Source: CAD feature listing. Evaluate the final solid. Frame: model axes, mm. A direction names the side the tool comes from. Give positions to 0.01 mm unless a question says otherwise; leave off trailing zeros. Write each loop counter-clockwise with the first axis right and the second up, starting at its lowest first coordinate (ties: lowest second). Pieces come first, ordered by that corner, then holes. Notation, with made-up numbers: (25.25, -37.75) -> (42.25, -37.75) arc R22 cw to (42.25, -25.75) -> close; hole circle Ø7 at (-29, 19.5). An arc over 180 degrees is marked (long way). Answer as a JSON object with one key per item and string values. Group by question number.
Item 1: Access query for faces 1 (the face through (0, 1, 13.5)), 2 (the face through (12.5, 1, -3)), 3 (the face through (13, 9, 0)), 4 (the face through (11.93, 10.01, 11.9)). Directions: +Z, -Z, +X, -X, +Y, -Y. A direction counts if a zero-diameter tool reaches every point of the face in a straight line with its end or side. Return the directions, or none.
Item 2: Section query C-C on x = -3.75. Return the cut outline in (y, z), plus the area to 3 significant figures.
Item 3: Section query D-D on z = -4.5. Return the cut outline in (x, y).
Item 4: First-contact query: pin 1 Ø0.6 at (y, z) = (1.5, -6.5) entering from -X; pin 2 Ø0.6 at (x, y) = (-1.5, 0.5) entering from -Z; pin 3 Ø2 at (y, z) = (0.5, -1.5) entering from +X; pin 4 Ø1.6 at (y, z) = (1.5, 10.5) entering from -X. Flat tips, straight axial feed; report the tip coordinate or a pass-through.
Item 5: Section query B-B on x = 7. Return the cut outline in (y, z).
Item 6: Section query A-A on z = 7.25. Return the cut outline in (x, y), plus the area to 3 significant figures.
Item 7: Ray query, probe 1 along X at (y, z) = (10, -5); probe 2 along Z at (x, y) = (4, 0.75); probe 3 along Z at (x, y) = (8.75, 1.5). Return the intervals inside material, ascending. Write a range as from..to.
from build123d import *

# Parameters (mm, degrees)
SKETCH1_W           = 29
SKETCH1_H           = 29
BOSS_EXTRUDE1_DEPTH = 11
CUT_EXTRUDE1_DEPTH  = 2
SKETCH3_W           = 29
SKETCH3_H           = 29
SKETCH3_W_2         = 25
SKETCH3_H_2         = 18
CUT_EXTRUDE2_DEPTH  = 2
SKETCH4_W           = 9.666666666
SKETCH4_H           = 4
BOSS_EXTRUDE2_DEPTH = 2


with BuildPart() as part:
    # Sketch1 → Boss-Extrude1 (new body)
    with BuildSketch(Plane(origin=(0, 0, 0), x_dir=(1, 0, 0), z_dir=(0, 1, 0))):
        Rectangle(SKETCH1_W, SKETCH1_H)
    extrude(amount=BOSS_EXTRUDE1_DEPTH)

    # Sketch2 → Cut-Extrude1 (cut)
    with BuildSketch(Plane(origin=(0, 11, 0), x_dir=(1, 0, 0), z_dir=(0, 1, 0))):
        with BuildLine():
            Line((-10.5, 17.5), (10.5, 17.5))
            ThreePointArc((10.5, 17.5), (15.449747468, 15.449747468), (17.5, 10.5))
            Line((17.5, 10.5), (17.5, -10.5))
            ThreePointArc((17.5, -10.5), (15.449747468, -15.449747468), (10.5, -17.5))
            Line((10.5, -17.5), (-10.5, -17.5))
            ThreePointArc((-10.5, -17.5), (-15.449747468, -15.449747468), (-17.5, -10.5))
            Line((-17.5, -10.5), (-17.5, 10.5))
            ThreePointArc((-17.5, 10.5), (-15.449747468, 15.449747468), (-10.5, 17.5))
        make_face()
        with BuildLine():
            Line((-10.5, 12.5), (10.5, 12.5))
            ThreePointArc((10.5, 12.5), (11.914213562, 11.914213562), (12.5, 10.5))
            Line((12.5, 10.5), (12.5, -10.5))
            ThreePointArc((12.5, -10.5), (11.914213562, -11.914213562), (10.5, -12.5))
            Line((10.5, -12.5), (-10.5, -12.5))
            ThreePointArc((-10.5, -12.5), (-11.914213562, -11.914213562), (-12.5, -10.5))
            Line((-12.5, -10.5), (-12.5, 10.5))
            ThreePointArc((-12.5, 10.5), (-11.914213562, 11.914213562), (-10.5, 12.5))
        make_face(mode=Mode.SUBTRACT)
    extrude(amount=-CUT_EXTRUDE1_DEPTH, mode=Mode.SUBTRACT)

    # Sketch3 → Cut-Extrude2 (cut)
    with BuildSketch(Plane(origin=(0, 0, 0), x_dir=(-1, 0, 0), z_dir=(0, -1, 0))):
        Rectangle(SKETCH3_W, SKETCH3_H)
        with Locations((0, 3.5)):
            Rectangle(SKETCH3_W_2, SKETCH3_H_2, mode=Mode.SUBTRACT)
    extrude(amount=-CUT_EXTRUDE2_DEPTH, mode=Mode.SUBTRACT)

    # Sketch4 → Boss-Extrude2 (add)
    with BuildSketch(Plane.XZ.offset(-2)):
        with Locations((0, 11.5)):
            Rectangle(SKETCH4_W, SKETCH4_H)
    extrude(amount=BOSS_EXTRUDE2_DEPTH)


solid = part.part
Worked answers:
{
 "1": {"face 1": "+Z, +X, -X, -Y", "face 2": "+Z, -Z, +X, -Y", "face 3": "+Y", "face 4": "+Z, +X, +Y"},
 "2": {"outline": "(0, -12.5) -> (2, -12.5) -> (2, -14.5) -> (9, -14.5) -> (9, -12.5) -> (11, -12.5) -> (11, 12.5) -> (9, 12.5) -> (9, 14.5) -> (2, 14.5) -> (2, 13.5) -> (0, 13.5) -> (0, 9.5) -> (2, 9.5) -> (2, 5.5) -> (0, 5.5) -> close", "area": "297 mm^2"},
 "3": {"outline": "(-14.5, 2) -> (-12.5, 2) -> (-12.5, 0) -> (12.5, 0) -> (12.5, 2) -> (14.5, 2) -> (14.5, 9) -> (12.5, 9) -> (12.5, 11) -> (-12.5, 11) -> (-12.5, 9) -> (-14.5, 9) -> close"},
 "4": {"pin 1": "x = -12.5", "pin 2": "z = -12.5", "pin 3": "x = 12.5", "pin 4": "x = -14.5"},
 "5": {"outline": "(0, -12.5) -> (2, -12.5) -> (2, -14.5) -> (9, -14.5) -> (9, -12.5) -> (11, -12.5) -> (11, 12.5) -> (9, 12.5) -> (9, 14.5) -> (2, 14.5) -> (2, 5.5) -> (0, 5.5) -> close"},
 "6": {"outline": "(-14.5, 2) -> (14.5, 2) -> (14.5, 9) -> (12.5, 9) -> (12.5, 11) -> (-12.5, 11) -> (-12.5, 9) -> (-14.5, 9) -> close", "area": "253 mm^2"},
 "7": {"probe 1": "-12.5..12.5", "probe 2": "-12.5..5.5, 9.5..13.5", "probe 3": "-12.5..5.5"}
}
